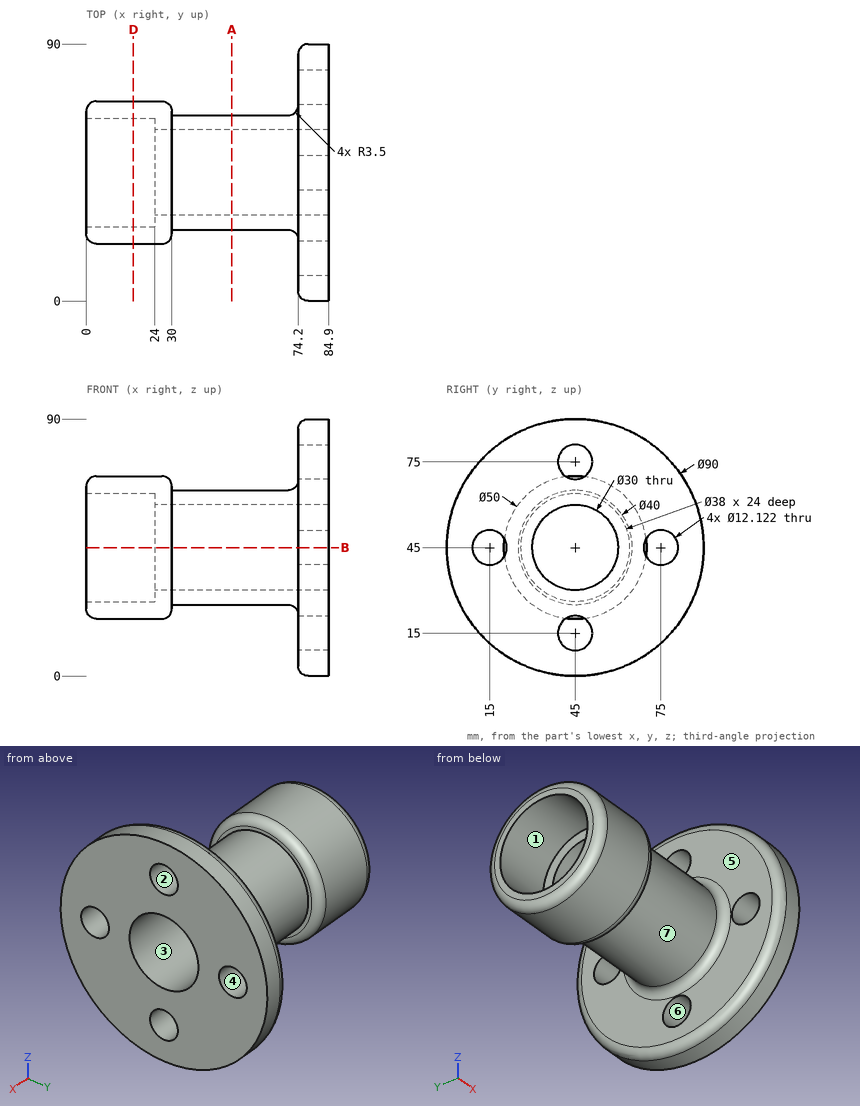
Design review of the part shown in the three views and the two pictorial views. Dimensions are in mm from the part's minimum x, y and z. A direction names the side the tool comes from. Give positions to 0.01 mm unless a question says otherwise; leave off trailing zeros. Write each loop counter-clockwise with the first axis right and the second up, starting at its lowest first coordinate (ties: lowest second). Pieces come first, ordered by that corner, then holes.
Item 1: Take a section at A-A (x = 51). Give the boundary of the cut face in (y, z), and give its area (3 significant figures).
Item 2: Take a section at D-D (x = 16.5). Give the boundary of the cut face in (y, z).
Item 3: Wall thickness on probe 1 along X at (y, z) = (81, 29); probe 2 along Y at (x, z) = (8.5, 51.5); probe 3 along X at (y, z) = (33, 65.5): over which ranges is each line inside the solid? List them lowest first.
Item 4: The part is to be moulded in two halves that separate along Z. For the marked faces 4, 5, 6 and 7, say which applies: +Z half, -Z half, draft (parallel to the pull), parting line (faces both ways), or undercut.
Item 5: Insertion check: P1, Ø9.5, axis at y = 45, z = 75, coming from the +X side; P2, Ø10, axis at x = 57.5, y = 24, coming from the +Z side; P3, Ø6, axis at x = 76.5, z = 73.5, coming from the -Y side; P4, Ø6, axis at x = 46, z = 61, coming from the +Y side. Each pin has a flat end and moves straight along its axis. Give the tip position at first contact, or say it passes through.
Item 6: Take a section at B-B (z = 45). Give the number of separate pieces and of enclosed holes in the cut face, and give its area (3 significant figures).
Item 7: Machinability: for the marked faces 1, 2 and 3, which of the approach directions +Z, -Z, +X, -X, +Y, -Y give a long, thin tool a straight path to every point of the face, cutting with its end or side? Answer none if there is none.
Established:
1. outline: circle Ø40 at (45, 45); hole circle Ø30 at (45, 45)
1. area: 550 mm2
2. outline: circle Ø50 at (45, 45); hole circle Ø38 at (45, 45)
3. probe 1: x = 74.2 to 84.9
3. probe 2: y = 20.86 to 27.15, 62.85 to 69.14
3. probe 3: x = 0.82 to 29.18, 74.2 to 84.9
4. face 4: undercut
4. face 5: draft
4. face 6: undercut
4. face 7: parting line
5. P1: passes through
5. P2: stops at z = 57
5. P3: stops at y = 8.02
5. P4: stops at y = 60.2
6. separate pieces: 4
6. enclosed holes: 0
6. area: 1,220 mm2
7. face 1: -X
7. face 2: +X
7. face 3: +X, -X
